Could you check a few things on this model? Use its own coordinates, in mm. Face numbers are marked on the shaded views. Give positions to 0.01 mm unless a question says otherwise; leave off trailing zeros. Write item = value, one per line.
from build123d import *

# Parameters (mm, degrees)
SKETCH1_R               = 5.08
EXTRUDE1_DEPTH          = 8.89
FILLET3_R               = 33.02
CUT_EXTRUDE1_START      = -4.4704
CUT_EXTRUDE1_DEPTH      = 4.4704
FILLET4_R               = 1.27
FILLET7_R               = 1.27
FILLET8_R               = 2.54
CUT_EXTRUDE4_START      = -2.4323391
CUT_EXTRUDE4_DEPTH      = 2.4323391
SKETCH7_R               = 9.5504
CUT_EXTRUDE5_DEPTH      = 127.908284031
CHAMFER1_SIZE           = 0.762
CHAMFER2_SIZE           = 1.27
CHAMFER2_SIZE2          = 1.513527063
CUT_EXTRUDE7_DEPTH      = 128.140710162
CUT_EXTRUDE7_DEPTH_BACK = 128.140710162


# Read off the part's stored shape, not the designer's step: Cut-Extrude4
with BuildPart() as part:
    # Sketch1 → Extrude1 (new body)
    with BuildSketch(Plane(origin=(0, 0, 0), x_dir=(1, 0, 0), z_dir=(0, 1, 0))):
        with BuildLine():
            Line((12.7, -74.068815454), (12.7, -71.528815454))
            Line((12.7, -71.528815454), (-19.839666339, -65.95654879))
            ThreePointArc((-19.839666339, -65.95654879), (-20.542938147, -65.783746069), (-21.214492201, -65.512697791))
            ThreePointArc((-21.214492201, -65.512697791), (-28.50851165, -65.065328333), (-33.972800967, -69.917585685))
            ThreePointArc((-33.972800967, -69.917585685), (-34.683898809, -71.939297222), (-34.925, -74.068815454))
            ThreePointArc((-34.925, -74.068815454), (-36.075887863, -78.537283812), (-39.242168201, -81.893832809))
            ThreePointArc((-39.242168201, -81.893832809), (-56.965393588, -89.848120853), (-76.2, -92.570864422))
            ThreePointArc((-76.2, -92.570864422), (-79.027338631, -97.190434), (-73.627220553, -97.606356539))
            ThreePointArc((-73.627220553, -97.606356539), (-50.892740286, -93.213306405), (-30.610706836, -82.042155988))
            ThreePointArc((-30.610706836, -82.042155988), (-21.042688621, -82.538730598), (-15.883271821, -74.465690454))
            Line((-15.883271821, -74.465690454), (12.7, -74.465690454))
            Line((12.7, -74.465690454), (12.7, -74.068815454))
        make_face()
        with Locations(Location((-25.4, -74.068815454, 0), (0, 0, 270))):
            Circle(SKETCH1_R, mode=Mode.SUBTRACT)
    extrude(amount=EXTRUDE1_DEPTH)

    # Fillet3
    fillet3_edges = [part.edges().sort_by_distance(p)[0] for p in [
        (-30.610706836, 4.445, 82.042155988),
    ]]
    fillet(fillet3_edges, radius=FILLET3_R)

    # Sketch4 → Cut-Extrude1 (cut)
    with BuildSketch(Plane(origin=(0, 8.89, 0), x_dir=(-1, 0, 0), z_dir=(0, 1, 0)).offset(CUT_EXTRUDE1_START)):
        with BuildLine():
            Line((17.299976936, 66.391458799), (17.620638494, 68.572711419))
            ThreePointArc((17.620638494, 68.572711419), (16.819560669, 78.20423392), (24.852605063, 83.578073247))
            Line((24.852605063, 83.578073247), (24.852605063, 89.837842614))
            Line((24.852605063, 89.837842614), (32.15380679, 89.837842614))
            Line((32.15380679, 89.837842614), (30.971364696, 81.794455907))
            ThreePointArc((30.971364696, 81.794455907), (33.355442096, 79.306808013), (34.698482461, 76.13372439))
            Line((34.698482461, 76.13372439), (35.179826108, 76.225066607))
            Line((35.179826108, 76.225066607), (37.134154695, 72.138642589))
            Line((37.134154695, 72.138642589), (28.798402731, 58.612170247))
            Line((28.798402731, 58.612170247), (17.299976936, 66.391458799))
        make_face()
    extrude(amount=CUT_EXTRUDE1_DEPTH, mode=Mode.SUBTRACT)

    # Fillet4
    fillet4_edges = [part.edges().sort_by_distance(p)[0] for p in [
        (-56.965393588, 8.89, 89.848120853),
        (-56.965393588, 0, 89.848120853),
        (-79.027338631, 8.89, 97.190434),
        (-79.027338631, 0, 97.190434),
        (-35.461557578, 8.89, 85.983630351),
        (-18.611736336, 0, 80.750514447),
        (-32.337042326, 0, 84.884424071),
        (-73.627220553, 4.445, 97.606356539),
        (-55.883733715, 8.89, 94.822561219),
        (-55.883733715, 0, 94.822561219),
        (-3.569833169, 0, 68.742682122),
        (-30.442750401, 0, 65.988203262),
        (-36.656296279, 8.89, 79.456958555),
        (-36.075887863, 0, 78.537283812),
        (-20.542938147, 0, 65.783746069),
    ]]
    fillet(fillet4_edges, radius=FILLET4_R)

    # Fillet7
    fillet7_edges = [part.edges().sort_by_distance(p)[0] for p in [
        (-2.299988468, 8.89, 68.960137126),
    ]]
    fillet(fillet7_edges, radius=FILLET7_R)

    # Fillet8
    # the kernel refuses this fillet: 2.54 mm, written as the material it takes off along each edge
    with BuildSketch(Plane(origin=(12.7, -4.085026029, 71.528815454), x_dir=(-0.9856523135338612, 0, -0.1687883788219644), z_dir=(0, 1, 0))) as fillet8_piece_1:
        with BuildLine():
            CenterArc((FILLET8_R * 0.843311185663, FILLET8_R), FILLET8_R, 189.717380318, 80.282619682)
            Line((-FILLET8_R * 0.142341127871, FILLET8_R * 0.831211621178), (0, 0))
            Line((0, 0), (FILLET8_R * 0.843311185663, 0))
        make_face()
    extrude(amount=17.060052058, mode=Mode.SUBTRACT)

    # Cut-Extrude4 outline → Cut-Extrude4 (cut)
    with BuildSketch(Plane.XY.offset(74.465690454).offset(CUT_EXTRUDE4_START)):
        with BuildLine():
            Line((12.7, 0), (12.7, 1.27))
            ThreePointArc((12.7, 1.27), (12.328025612, 0.371974388), (11.43, 0))
            Line((11.43, 0), (12.7, 0))
        make_face()
        with BuildLine():
            ThreePointArc((11.43, 8.89), (12.328025612, 8.518025612), (12.7, 7.62))
            Line((12.7, 7.62), (12.7, 8.89))
            Line((12.7, 8.89), (11.43, 8.89))
        make_face()
    extrude(amount=CUT_EXTRUDE4_DEPTH, mode=Mode.SUBTRACT)

    # Sketch7 → Cut-Extrude5 (cut, through all)
    with BuildSketch(Plane(origin=(0, 4.4196, 0), x_dir=(-1, 0, 0), z_dir=(0, 1, 0))):
        with Locations((25.4, 74.068815454)):
            Circle(SKETCH7_R)
    extrude(amount=CUT_EXTRUDE5_DEPTH, mode=Mode.SUBTRACT)

    # Chamfer1
    chamfer1_edges = [part.edges().sort_by_distance(p)[0] for p in [
        (-25.4, 0, 68.988815454),
    ]]
    chamfer(chamfer1_edges, length=CHAMFER1_SIZE)

    # Chamfer2
    chamfer2_edges = [part.edges().sort_by_distance(p)[0] for p in [
        (-25.4, 4.4196, 68.988815454),
    ]]
    chamfer2_side = [part.faces().sort_by_distance(p)[0] for p in [
        (-18.616859876, 4.4196, 66.448687097),
    ]]
    chamfer(chamfer2_edges, length=CHAMFER2_SIZE, length2=CHAMFER2_SIZE2, reference=chamfer2_side[0])

    # Sketch9 → Cut-Extrude7 (cut, two sides: drawn at the far end of the back side and taken through both)
    with BuildSketch(Plane(origin=(0, 8.89, 0), x_dir=(-1, 0, 0), z_dir=(0, 1, 0)).offset(-CUT_EXTRUDE7_DEPTH_BACK)):
        Polygon((0.79375, 73.671940454), (1.5875, 74.465690454), (0, 74.465690454), align=None)
        Polygon((2.38125, 73.671940454), (3.175, 74.465690454), (1.5875, 74.465690454), align=None)
        Polygon((3.96875, 73.671940454), (4.7625, 74.465690454), (3.175, 74.465690454), align=None)
        Polygon((11.90625, 73.671940454), (12.7, 74.465690454), (11.1125, 74.465690454), align=None)
        Polygon((13.485174901, 73.680515552), (14.270349802, 74.465690454), (12.7, 74.465690454), align=None)
        Polygon((10.31875, 73.671940454), (11.1125, 74.465690454), (9.525, 74.465690454), align=None)
        Polygon((8.73125, 73.671940454), (9.525, 74.465690454), (7.9375, 74.465690454), align=None)
        Polygon((7.14375, 73.671940454), (7.9375, 74.465690454), (6.35, 74.465690454), align=None)
        Polygon((5.55625, 73.671940454), (6.35, 74.465690454), (4.7625, 74.465690454), align=None)
        Polygon((15.064099802, 73.671940454), (15.857849802, 74.465690454), (14.270349802, 74.465690454), align=None)
        Polygon((-0.79375, 73.671940454), (0, 74.465690454), (-1.5875, 74.465690454), align=None)
        Polygon((-2.38125, 73.671940454), (-1.5875, 74.465690454), (-3.175, 74.465690454), align=None)
        Polygon((-3.96875, 73.671940454), (-3.175, 74.465690454), (-4.7625, 74.465690454), align=None)
        Polygon((-5.55625, 73.671940454), (-4.7625, 74.465690454), (-6.35, 74.465690454), align=None)
        Polygon((-7.14375, 73.671940454), (-6.35, 74.465690454), (-7.9375, 74.465690454), align=None)
        Polygon((-8.73125, 73.671940454), (-7.9375, 74.465690454), (-9.525, 74.465690454), align=None)
        Polygon((-10.31875, 73.671940454), (-9.525, 74.465690454), (-11.1125, 74.465690454), align=None)
    extrude(amount=CUT_EXTRUDE7_DEPTH + CUT_EXTRUDE7_DEPTH_BACK, mode=Mode.SUBTRACT)


solid = part.part
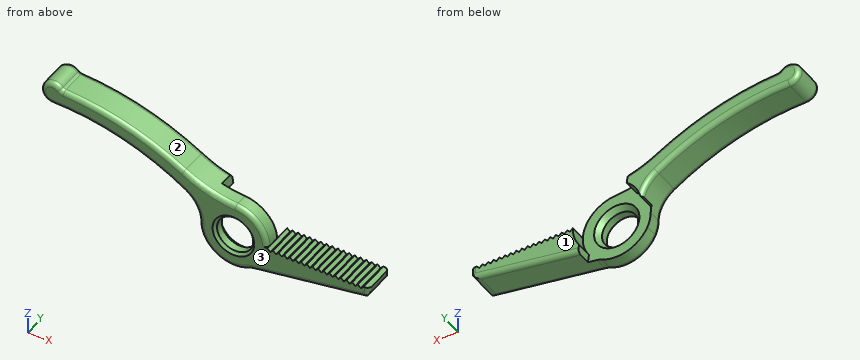
1. Thinking about a two-plate mould opening in Y: for the marked faces 1, 2 and 3, which applies, pulls with the +Y half, pulls with the -Y half, needs draft (parallel to the pull), parting line crosses it, or undercut?
Filled sheet:
face_1 = pulls with the +Y half
face_2 = needs draft
face_3 = pulls with the -Y half
2. I need wall thicknesses on line 1 (Z direction, x = -25.4, y = 1.65); line 2 (Z direction, x = -21, y = 3.5); line 3 (Z direction, x = -13, y = 5.25). Which ranges of each line are inside material? Lowest first, please.
Filled sheet:
line_1 = 64.54 to 68.99, 79.15 to 83.61
line_2 = 65.61 to 70.64, 77.5 to 82.52
line_3 = 67.13 to 74.17
3. For pin 1 (1.5 mm diameter, centred on x = -30.5, y = 3, fed in from +Z); pin 2 (1.3 mm diameter, centred on x = 11.5, y = 6.5, fed in from +Z); pin 3 (1 mm diameter, centred on x = -35, y = 4.5, fed in from +Z), each with a flat end and sliding along its axis, tell me the tip position at first contact or that it passes through.
Filled sheet:
pin_1 = 84.58
pin_2 = 74.47
pin_3 = 86
